Autodesk Inventor part; units mm, degrees
ref_plane "XZ Plane" through (0, 0, 0) normal (0, 1, 0) x (-1, 0, 0)
ref_plane "XY Plane" through (0, 0, 0) normal (0, 0, 1) x (1, 0, 0)
sketch "Sketch1" plane through (0, 0, 0) normal (1, 0, 0) x (0, 1, 0)
  line L0 (-5, 5) -> (5, 5)
  line L1 (5, 5) -> (5, -5)
  line L2 (5, -5) -> (-5, -5)
  line L3 (-5, -5) -> (-5, 5)
  line L4 (-5, 5) -> (5, -5) construction
  line L5 (5, 5) -> (-5, -5) construction
  line L6 (-4, 4) -> (4, 4)
  line L7 (4, 4) -> (4, -4)
  line L8 (4, -4) -> (-4, -4)
  line L9 (-4, -4) -> (-4, 4)
  line L10 (-4, 4) -> (4, -4) construction
  line L11 (4, 4) -> (-4, -4) construction
  point P0 (0, 0)
  dimension "d0" = 10
  dimension "d1" = 10
  dimension "d2" = 8
  dimension "d3" = 8
extrude "Extrusion1" add sketch "Sketch1" along normal mid plane 350
sketch "Sketch2" plane through (-175, 5, 5) normal (0, 1, 0) x (1, 0, 0)
  circle A0 centre (6, 5) radius 2.6
  line L0 (26, 5) -> (41, 5) construction
  line L1 (26, 2.4) -> (41, 2.4)
  line L2 (41, 7.6) -> (26, 7.6)
  arc A1 (26, 7.6) -> (26, 2.4) centre (26, 5) ccw
  arc A2 (41, 2.4) -> (41, 7.6) centre (41, 5) ccw
  line L3 (0, 0) -> (0, 10)
  circle A3 centre (82, 5) radius 2.6
  circle A4 centre (144, 5) radius 2.6
  point P0 (175, 5)
  point P1 (33.5, 5)
  dimension "d6" = 5.2
  dimension "d7" = 6
  dimension "d8" = 20
  dimension "d9" = 15
  dimension "d13" = 62
  dimension "d14" = 31
extrude "Extrusion2" cut sketch "Sketch2" against normal blind 100
mirror "Mirror1" about plane through (0, 0, 0) normal (1, 0, 0) of "Extrusion2"
properties part number "holder_bar"
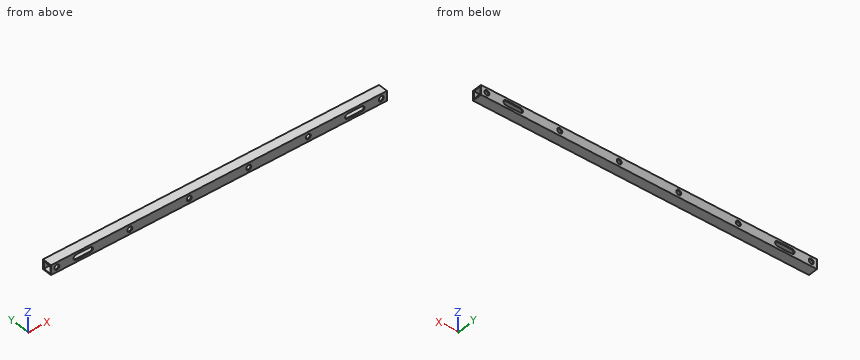
Geometry check sheet. Reference: the model listing, model coordinates, mm. Give positions to 0.01 mm unless a question says otherwise; leave off trailing zeros. Order: outer loops, then holes, each group sorted by start corner. A loop starts at its lowest first (then second) coordinate and runs counter-clockwise, first axis right, second up. Notation, with made-up numbers: (9.5, -3) - (13.5, -3) arc R26 ccw to (13.5, 27) - close; hole circle Ø3 at (46.5, 80). An arc over 180 degrees is marked (long way). Write item = value, one per line. Start each with the question number.
1) Section check A-A (y = -0.25). Enter the section's corners in (x, z).
2) Section check C-C (z = 0). Count the separate pieces of the cut face and the enclosed holes in it, then the cut area to 3 significant figures.
3) Scan lines: L1, parallel to Z at x = 169, y = -4.6; L2, parallel to Y at x = 52, z = 2.75. Record each from-to range of solid material in increasing order.
4) Section check B-B (x = -39). Enter the section's corners in (y, z), then the cut area to 3 significant figures.
Geometry check:
q1.outline = (-175, -5) - (175, -5) - (175, -4) - (-175, -4) - close; (-175, 4) - (175, 4) - (175, 5) - (-175, 5) - close
q2.separate_pieces = 18
q2.enclosed_holes = 0
q2.area = 557 mm2
q3.L1 = -5 to -2.6, 2.6 to 5
q3.L2 = -5 to -4, 4 to 5
q4.outline = (-5, -5) - (5, -5) - (5, 5) - (-5, 5) - close; hole (-4, -4) - (4, -4) - (4, 4) - (-4, 4) - close
q4.area = 36.0 mm2
